Can you work these out from the model? Positions are in its coordinate system, mm. Face numbers are marked on the shaded views. A direction names the side the tool comes from. Coordinates: 2 decimals unless noted, no trailing zeros. Write each loop counter-clockwise with the first axis right and the second up, starting at its lowest first coordinate (ties: lowest second). Pieces come first, ordered by that corner, then holes. Notation, with made-up numbers: (9, -25.5) - (41, -25.5) arc R28 ccw to (41, -6.5) - close; hole circle Ø6 at (-1.5, 62). An arc over 180 degrees is marked (long way). Use one line per item in the form item = value. Start each with the question number.
(1) On a 3-axis mill with a long thin cutter (end or side, diameter ignored), from which of +Z, -Z, +X, -X, +Y, -Y can I reach the whole of each face in a straight line? I mean the marked faces 1, 2 and 3. Say none if no direction works.
(2) For pin 1 Ø1.6 at (y, z) = (-9.5, 1.5) entering from +X; pin 2 Ø1.1 at (y, z) = (4.5, 2) entering from -X (3 decimals); pin 3 Ø1 at (x, z) = (20.5, 2.5) entering from +Y; pin 4 Ø1 at (x, z) = (-21, 1.5) entering from -Y, each with a flat end and sliding along its axis, tell me the tip position at first contact or that it passes through.
(3) If I drill on probe 1 along X at (y, z) = (-13, 2.65), over which ranges is the centre line in solid material (lowest first)? Write a range as from..to.
(4) If we section it at B-B on y = -10.75: Please give me the cut outline in (x, z) (3 decimals), then the cut area to 3 significant figures.
(5) If we section it at A-A on z = 0.45: Please give me the cut outline in (x, y) (3 decimals).
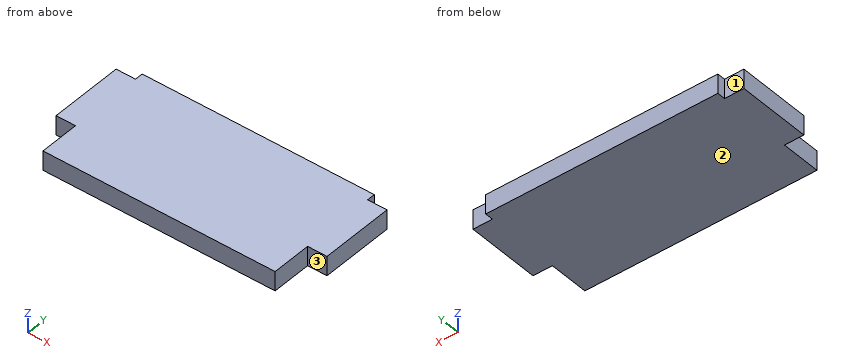
```python
from build123d import *

# Parameters (mm, degrees)
SKETCH1_W           = 3.175
SKETCH1_H           = 12
SKETCH1_H_2         = 18
BOSS_EXTRUDE1_DEPTH = 3.175
SKETCH2_W           = 32.65
SKETCH2_H           = 2
BOSS_EXTRUDE2_DEPTH = 3.175
SKETCH3_W           = 3.175
SKETCH3_H           = 1.331730769
CUT_EXTRUDE2_DEPTH  = 10
SKETCH5_W           = 5.35
SKETCH5_H           = 2
BOSS_EXTRUDE5_DEPTH = 3.175


with BuildPart() as part:
    # Sketch1 → Boss-Extrude1 (new body)
    with BuildSketch(Plane.XY):
        Polygon((19, 5.331730769), (-19, 12.5), (-19, 10), (-19, -8), (-19, -12.5), (19, -12.5), (19, -8), (19, 4), align=None)
        with Locations((20.5875, -2)):
            Rectangle(SKETCH1_W, SKETCH1_H)
        with Locations((-20.5875, 1)):
            Rectangle(SKETCH1_W, SKETCH1_H_2)
    extrude(amount=BOSS_EXTRUDE1_DEPTH)

    # Sketch2 → Boss-Extrude2 (add)
    with BuildSketch(Plane.XY.offset(3.175)):
        with Locations((2.675, -13.5)):
            Rectangle(SKETCH2_W, SKETCH2_H)
    extrude(amount=-BOSS_EXTRUDE2_DEPTH)

    # Sketch3 → Cut-Extrude2 (cut)
    with BuildSketch(Plane.XY.offset(3.175)):
        with Locations((-20.5875, 4.665865384)):
            Rectangle(SKETCH3_W, SKETCH3_H)
        Polygon((-19, 5.331730769), (-19, 9.853630911), (-19, 10), (-22.175, 10), (-22.175, 5.331730769), align=None)
        Polygon((-19, 10), (-19, 9.853630911), (-19, 5.331730769), (19, 5.331730769), (-11.823223146, 11.146182403), (-19, 11.146182403), align=None)
        Polygon((-19, 12.5), (-19, 11.146182403), (-11.823223146, 11.146182403), align=None)
    extrude(amount=-CUT_EXTRUDE2_DEPTH, mode=Mode.SUBTRACT)

    # Sketch5 → Boss-Extrude5 (add)
    with BuildSketch(Plane.XY.offset(3.175)):
        with Locations((-16.325, -13.5)):
            Rectangle(SKETCH5_W, SKETCH5_H)
    extrude(amount=-BOSS_EXTRUDE5_DEPTH)


solid = part.part
```
Reported:
q1.face_1 = +Z, -Z, -X, +Y
q1.face_2 = -Z, +X, -X, +Y, -Y
q1.face_3 = +Z, -Z, +X, -Y
q2.pin_1 = 19
q2.pin_2 = -22.175
q2.pin_3 = 4
q2.pin_4 = -8
q3.probe_1 = -19..19
q4.outline = (-19, 0) - (19, 0) - (19, 3.175) - (-19, 3.175) - close
q4.area = 121 mm2
q5.outline = (-22.175, -8) - (-19, -8) - (-19, -14.5) - (19, -14.5) - (19, -8) - (22.175, -8) - (22.175, 4) - (19, 4) - (19, 5.332) - (-19, 5.332) - (-19, 4) - (-22.175, 4) - close
